```python
from build123d import *

# Parameters (mm, degrees)
SKETCH1_W           = 37.16
SKETCH1_H           = 54.67
BOSS_EXTRUDE1_DEPTH = 3.65
FILLET1_R           = 3
FILLET2_R           = 2
SKETCH2_R           = 0.900344027
BOSS_EXTRUDE2_DEPTH = 3


with BuildPart() as part:
    # Sketch1 → Boss-Extrude1 (new, symmetric)
    with BuildSketch(Plane.XY):
        Rectangle(SKETCH1_W, SKETCH1_H)
    extrude(amount=BOSS_EXTRUDE1_DEPTH, both=True)

    # Fillet1
    fillet1_edges = [part.edges().sort_by_distance(p)[0] for p in [
        (-18.58, 0, 3.65),
        (18.58, 0, 3.65),
        (-18.58, 0, -3.65),
        (18.58, 0, -3.65),
    ]]
    fillet(fillet1_edges, radius=FILLET1_R)

    # Fillet2
    fillet2_edges = [part.edges().sort_by_distance(p)[0] for p in [
        (-18.58, 27.335, 0),
        (0, 27.335, -3.65),
        (0, 27.335, 3.65),
        (18.58, 27.335, 0),
        (17.701320344, 27.335, 2.771320344),
        (17.701320344, 27.335, -2.771320344),
        (-17.701320344, 27.335, 2.771320344),
        (-17.701320344, 27.335, -2.771320344),
    ]]
    fillet(fillet2_edges, radius=FILLET2_R)

    # Sketch2 → Boss-Extrude2 (add)
    with BuildSketch(Plane(origin=(0, 27.335, 0), x_dir=(1, 0, 0), z_dir=(0, 1, 0))):
        with Locations(Location((-1, 0, 0), (0, 0, 90))):
            Circle(SKETCH2_R)
        with Locations(Location((1, 0, 0), (0, 0, 90))):
            Circle(SKETCH2_R)
    extrude(amount=BOSS_EXTRUDE2_DEPTH)


solid = part.part
```
Read the model definition and answer for the solid it produces. Units are mm, in the model's axes. A direction names the side the tool comes from. Coordinates: 2 decimals unless noted, no trailing zeros. Write each loop counter-clockwise with the first axis right and the second up, starting at its lowest first coordinate (ties: lowest second). Pieces come first, ordered by that corner, then holes. Notation, with made-up numbers: (10.5, -7.75) -> (14.5, -7.75) arc R24 ccw to (14.5, 3.25) -> close; hole circle Ø6 at (-12.5, -5). An arc over 180 degrees is marked (long way). Answer as a JSON object with one key per item and string values.
Q1. The part is cut by section A-A on z = 0. Give the vertices of the cut face in (x, y) (3 decimals).
The answers:
{"outline": "(-18.58, -27.335) -> (18.58, -27.335) -> (18.58, 25.335) arc R2 ccw to (16.58, 27.335) -> (1.9, 27.335) -> (1.9, 30.335) -> (0.1, 30.335) -> (0.1, 27.335) -> (-0.1, 27.335) -> (-0.1, 30.335) -> (-1.9, 30.335) -> (-1.9, 27.335) -> (-16.58, 27.335) arc R2 ccw to (-18.58, 25.335) -> close"}
Q2. A tool of negligible diameter and unlimited length cuts with its end or side. For faces 1 (the flat face through (18.58, -1, 0)), 2 (the cylindrical face through (-1.893, 28.814, 0.117)), from which of +Z, -Z, +X, -X, +Y, -Y can it reach the whole face along a straight path? Write none if from no direction.
The answers:
{"face 1": "+Z, -Z, +X, +Y, -Y", "face 2": "+Y"}
Q3. The part is cut by section C-C on y = -23. Give the vertices of the cut face in (x, z), then the cut area to 3 significant figures.
The answers:
{"outline": "(-18.58, -0.65) arc R3 ccw to (-15.58, -3.65) -> (15.58, -3.65) arc R3 ccw to (18.58, -0.65) -> (18.58, 0.65) arc R3 ccw to (15.58, 3.65) -> (-15.58, 3.65) arc R3 ccw to (-18.58, 0.65) -> close", "area": "264 mm2"}
Q4. The part is cut by section B-B on x = -1. Give the vertices of the cut face in (y, z) (3 decimals).
The answers:
{"outline": "(-27.335, -3.65) -> (25.335, -3.65) arc R2 ccw to (27.335, -1.65) -> (27.335, -0.9) -> (30.335, -0.9) -> (30.335, 0.9) -> (27.335, 0.9) -> (27.335, 1.65) arc R2 ccw to (25.335, 3.65) -> (-27.335, 3.65) -> close"}
Q5. Determine the mould class of faces 3 (the cylindrical face through (0.218, 26.734, -3.08)), 4 (the cylindrical face through (0.107, 28.814, 0.117)), 5 (the cylindrical face through (-18.01, 26.734, -0.009)) for opening direction X: pulls with the +X half, pulls with the -X half, needs draft (parallel to the pull), parting line crosses it, or undercut.
The answers:
{"face 3": "needs draft", "face 4": "undercut", "face 5": "pulls with the -X half"}
Q6. Consider line 1 (Y direction, x = 4, z = -1.5) (3 decimals); line 2 (X direction, y = -18, z = 0.75); line 3 (X direction, y = -5.5, z = 2.25). Determine where each line is inside the solid, lowest interval first. Write a range as [from, to].
The answers:
{"line 1": "y = [-27.335, 27.335]", "line 2": "x = [-18.58, 18.58]", "line 3": "x = [-18.12, 18.12]"}
Q7. Flat-ended cylindrical pins translate along their axes: pin 1 Ø2 at (x, z) = (14, 1) entering from +Y (3 decimals); pin 2 Ø1 at (y, z) = (16, 1.5) entering from -X. Find the tip coordinate at first contact, or state that the pin passes through.
The answers:
{"pin 1": "stops at y = 27.335", "pin 2": "stops at x = -18.56"}
